from build123d import *

# Parameters (mm, degrees)
SKETCH_1_R          = 1
EXTRUDE_1_DEPTH     = 2
SKETCH_2_W          = 3
SKETCH_2_H          = 15
EXTRUDE_2_DEPTH     = 25
FILLET_1_R          = 7.5
SKETCH_3_R          = 2.1
CUT_EXTRUDE_1_DEPTH = 15
FILLET_2_R          = 2


with BuildPart() as part:
    # 草图1 → 凸台-拉伸1 (new body)
    with BuildSketch(Plane.XY):
        Polygon((1.466666667, 10.933333333), (13.466666667, 10.933333333), (13.466666667, -9.066666667), (-31.533333333, -9.066666667), (-31.533333333, 10.933333333), (-19.533333333, 10.933333333), (-19.533333333, 5.933333333), (1.466666667, 5.933333333), align=None)
        with Locations((-30.333333333, 9.733333333)):
            Circle(SKETCH_1_R, mode=Mode.SUBTRACT)
        with Locations((-30.333333333, -7.866666667)):
            Circle(SKETCH_1_R, mode=Mode.SUBTRACT)
        with Locations((12.266666667, 9.733333333)):
            Circle(SKETCH_1_R, mode=Mode.SUBTRACT)
        with Locations((12.266666667, -7.866666667)):
            Circle(SKETCH_1_R, mode=Mode.SUBTRACT)
    extrude(amount=EXTRUDE_1_DEPTH)

    # 草图2 → 凸台-拉伸2 (add)
    with BuildSketch(Plane.XY.offset(2)):
        with Locations((-12.533333333, -1.566666667)):
            Rectangle(SKETCH_2_W, SKETCH_2_H)
        with Locations((-5.533333333, -1.566666667)):
            Rectangle(SKETCH_2_W, SKETCH_2_H)
    extrude(amount=EXTRUDE_2_DEPTH)

    # 圆角1
    fillet_1_edges = [part.edges().sort_by_distance(p)[0] for p in [
        (-5.533333333, -9.066666667, 27),
        (-12.533333333, -9.066666667, 27),
        (-5.533333333, 5.933333333, 27),
        (-12.533333333, 5.933333333, 27),
    ]]
    fillet(fillet_1_edges, radius=FILLET_1_R - 0.0001)  # a hair under: the kernel refuses the full size

    # 草图3 → 切除-拉伸1 (cut)
    with BuildSketch(Plane(origin=(-4.033333333, 0, 0), x_dir=(0, 0, -1), z_dir=(1, 0, 0))):
        with Locations(Location((-19.5, -1.566666667, 0), (0, 0, 90))):
            Circle(SKETCH_3_R)
    extrude(amount=-CUT_EXTRUDE_1_DEPTH, mode=Mode.SUBTRACT)

    # 圆角2
    fillet_2_edges = [part.edges().sort_by_distance(p)[0] for p in [
        (-14.033333333, -1.566666667, 2),
        (-4.033333333, -1.566666667, 2),
    ]]
    fillet(fillet_2_edges, radius=FILLET_2_R)


solid = part.part
For this review, take the finished solid that the model builds, in its own axes (mm). A direction names the side the tool comes from. Round coordinates to 2 decimals unless told otherwise and drop trailing zeros. Order: outer loops, then holes, each group sorted by start corner. A loop starts at its lowest first (then second) coordinate and runs counter-clockwise, first axis right, second up. Notation, with made-up numbers: (77, -36.75) -> (96, -36.75) arc R16 cw to (96, -5.75) -> close; hole circle Ø5 at (30, 48). An arc over 180 degrees is marked (long way). Write item = value, one per line. Start each with the question number.
1) Insertion check: pin 1 (4.5 mm diameter, centred on y = -3, z = 15, fed in from -X); pin 2 (15.5 mm diameter, centred on x = -10.5, z = 11, fed in from +Y); pin 3 (2 mm diameter, centred on y = -4, z = 19, fed in from +X). Each pin has a flat end and moves straight along its axis. Give the tip position at first contact, or say it passes through.
2) Take a section at A-A on y = 7.25. State the section outline as (x, z) points, plus the area to 3 significant figures.
3) Tool access review of faces 1 (the face through (-11.033, -2, 14)), 2 (the face through (7, 10.933, 1)), 3 (the face through (6, 1, 2)): name each direction out of +Z, -Z, +X, -X, +Y, -Y from which nothing blocks a thin tool from reaching the whole face with its end or side.
4) Take a section at D-D on y = 3. State the section outline as (x, z) points.
5) To check wall thickness, follow line 1 (X direction, y = 5.75, z = 17.5); line 2 (Z direction, x = -16.5, y = -2.5); line 3 (X direction, y = -3, z = 3.5). State the ranges of each line that lie inside material, in increasing order. Write a range as from..to.
6) Take a section at C-C on x = 0. State the section outline as (y, z) points, plus the area to 3 significant figures.
7) The part is to be moulded in two halves that separate along Y. For faces 4 (the face through (-6.8, 5.933, 9.6)), 5 (the face through (-30.464, -6.875, 0.986)), 6 (the face through (-19.533, 8, 1)), say which applies: +Y half, -Y half, draft (parallel to the pull), parting line (faces both ways), or undercut.
8) Take a section at B-B on z = 14.75. State the section outline as (x, y) points.
Verdict:
q1.pin_1 = -14.03
q1.pin_2 = 5.93
q1.pin_3 = -4.03
q2.outline = (-31.53, 0) -> (-19.53, 0) -> (-19.53, 2) -> (-31.53, 2) -> close; (1.47, 0) -> (13.47, 0) -> (13.47, 2) -> (1.47, 2) -> close
q2.area = 48.0 mm2
q3.face_1 = +Z, +Y, -Y
q3.face_2 = +Z, -Z, +X, -X, +Y
q3.face_3 = +Z, +X, +Y, -Y
q4.outline = (-31.53, 0) -> (13.47, 0) -> (13.47, 2) -> (-2.03, 2) arc R2 cw to (-4.03, 4) -> (-4.03, 25.45) -> (-7.03, 25.45) -> (-7.03, 2) -> (-11.03, 2) -> (-11.03, 25.45) -> (-14.03, 25.45) -> (-14.03, 4) arc R2 cw to (-16.03, 2) -> (-31.53, 2) -> close
q5.line_1 = -14.03..-11.03, -7.03..-4.03
q5.line_2 = 0..2
q5.line_3 = -14.1..-11.03, -7.03..-3.97
q6.outline = (-9.07, 0) -> (5.93, 0) -> (5.93, 2) -> (-9.07, 2) -> close
q6.area = 30.0 mm2
q7.face_4 = +Y half
q7.face_5 = undercut
q7.face_6 = draft
q8.outline = (-14.03, -9.07) -> (-11.03, -9.07) -> (-11.03, 5.93) -> (-14.03, 5.93) -> close; (-7.03, -9.07) -> (-4.03, -9.07) -> (-4.03, 5.93) -> (-7.03, 5.93) -> close
